Input: part model. Units: mm. Frame: model coordinates. A direction names the side the tool comes from. Give positions to 0.01 mm unless a question says otherwise; leave off trailing zeros. Write each loop counter-clockwise with the first axis right and the second up, starting at its lowest first coordinate (ties: lowest second). Pieces come first, ordered by that corner, then holes. Notation, with made-up numbers: (-19.5, 18) - (8.5, 18) arc R28 cw to (8.5, 38) - close; hole circle Ø11 at (52, 28). An arc over 180 degrees is marked (long way). Answer as CSV lines item,"result".
```python
from build123d import *

# Parameters (mm, degrees)
SKETCH1_R           = 15
BOSS_EXTRUDE1_DEPTH = 3
SKETCH2_W           = 3
SKETCH2_H           = 17
BOSS_EXTRUDE2_DEPTH = 15
CUT_EXTRUDE1_DEPTH  = 25
SKETCH4_W           = 20
SKETCH4_H           = 6
CUT_EXTRUDE2_DEPTH  = 11
CUT_EXTRUDE3_DEPTH  = 25


with BuildPart() as part:
    # Sketch1 → Boss-Extrude1 (new body)
    with BuildSketch(Plane(origin=(0, 0, 0), x_dir=(1, 0, 0), z_dir=(0, 1, 0))):
        Circle(SKETCH1_R)
    extrude(amount=BOSS_EXTRUDE1_DEPTH)

    # Sketch2 → Boss-Extrude2 (add)
    with BuildSketch(Plane(origin=(0, 3, 0), x_dir=(1, 0, 0), z_dir=(0, 1, 0))):
        with Locations((-7.5, 0)):
            Rectangle(SKETCH2_W, SKETCH2_H)
        with Locations((7.5, 0)):
            Rectangle(SKETCH2_W, SKETCH2_H)
    extrude(amount=BOSS_EXTRUDE2_DEPTH)

    # Sketch3 → Cut-Extrude1 (cut, through all)
    with BuildSketch(Plane.ZY.offset(9)):
        with BuildLine():
            Line((-8.5, 9.4), (-8.5, 18))
            Line((-8.5, 18), (8.5, 18))
            Line((8.5, 18), (8.5, 9.4))
            ThreePointArc((8.5, 9.4), (0, 17.9), (-8.5, 9.4))
        make_face()
    extrude(amount=-CUT_EXTRUDE1_DEPTH, mode=Mode.SUBTRACT)

    # Sketch4 → Cut-Extrude2 (cut)
    with BuildSketch(Plane(origin=(0, 0, 0), x_dir=(-1, 0, 0), z_dir=(0, -1, 0))):
        Rectangle(SKETCH4_W, SKETCH4_H)
    extrude(amount=-CUT_EXTRUDE2_DEPTH, mode=Mode.SUBTRACT)

    # Sketch5 → Cut-Extrude3 (cut, through all)
    with BuildSketch(Plane.ZY.offset(9)):
        with BuildLine():
            Line((3, 11), (-3, 11))
            ThreePointArc((-3, 11), (0, 14), (3, 11))
        make_face()
    extrude(amount=-CUT_EXTRUDE3_DEPTH, mode=Mode.SUBTRACT)


solid = part.part
```
Item 1: Cut plane C-C on y = 5.5. Return the cut outline in (x, z).
The answers:
outline,"(-9, -8.5) - (-6, -8.5) - (-6, -3) - (-9, -3) - close; (-9, 3) - (-6, 3) - (-6, 8.5) - (-9, 8.5) - close; (6, -8.5) - (9, -8.5) - (9, -3) - (6, -3) - close; (6, 3) - (9, 3) - (9, 8.5) - (6, 8.5) - close"
Item 2: Mould query, pull axis X, two halves, no side actions, for faces 5 (the face through (-9, 10, -4)), 6 (the face through (0, 0, -4)), 7 (the face through (6, 10, -4)). Classes: +X half, -X half, draft (parallel to the pull), parting line (faces both ways), or undercut.
The answers:
face 5,"-X half"
face 6,"draft"
face 7,"undercut"
Item 3: Contact query for flat-ended pins moving along their axis: pin 1 (6 mm diameter, centred on x = 12, z = 10, fed in from +Y); pin 2 (0.9 mm diameter, centred on x = -7.5, y = 7.5, fed in from -Z); pin 3 (10 mm diameter, centred on x = 1.5, y = 11.5, fed in from +Z); pin 4 (2 mm diameter, centred on x = 3.5, z = 1, fed in from +Y). Output: stop coordinate, or through.
The answers:
pin 1,"y = 3"
pin 2,"z = -8.5"
pin 3,"z = 8.5"
pin 4,"through"
Item 4: Reachability of faces 1 (the face through (-2, 2, -3)), 2 (the face through (-6, 10, -4)), 3 (the face through (-8, 6, 8.5)), 4 (the face through (10, 1, 0)) from +Z, -Z, +X, -X, +Y, -Y: full face, straight path, thin tool, end or side. Return the list, or none.
The answers:
face 1,"-Y"
face 2,"+Z, -Z, +Y"
face 3,"+Z, +X, -X, +Y"
face 4,"+Y, -Y"
Item 5: Cut plane D-D on y = 1. Return the cut outline in (x, z).
The answers:
outline,"circle Ø30 at (0, 0); hole (-10, -3) - (10, -3) - (10, 3) - (-10, 3) - close"
Item 6: Cut plane A-A on x = 0. Return the cut outline in (y, z), plus the area to 3 significant figures.
The answers:
outline,"(0, -15) - (3, -15) - (3, -3) - (0, -3) - close; (0, 3) - (3, 3) - (3, 15) - (0, 15) - close"
area,"72.0 mm²"
Item 7: Ray query, line 1 (X direction, y = 11.5, z = 7.5); line 2 (Z direction, x = -8.5, y = 9.75); line 3 (Y direction, x = -4.5, z = -10.75). Return the intervals inside material, ascending. Write a range as from..to.
The answers:
line 1,"-9..-6, 6..9"
line 2,"-8.49..-3, 3..8.49"
line 3,"0..3"
Item 8: Cut plane B-B on z = 0. Return the cut outline in (x, y).
The answers:
outline,"(-15, 0) - (-10, 0) - (-10, 3) - (-15, 3) - close; (-9, 14) - (-6, 14) - (-6, 17.9) - (-9, 17.9) - close; (6, 14) - (9, 14) - (9, 17.9) - (6, 17.9) - close; (10, 0) - (15, 0) - (15, 3) - (10, 3) - close"
